Can you work these out from the model? Positions are in its coordinate system, mm. A direction names the side the tool comes from. Give positions to 0.01 mm unless a question says otherwise; leave off trailing zeros. Order: outer loops, then holes, each group sorted by start corner. A loop starts at its lowest first (then second) coordinate and runs counter-clockwise, first axis right, second up. Notation, with made-up numbers: (13.25, 55) -> (17.25, 55) arc R20 cw to (17.25, 80) -> close; hole circle Ø2 at (2, 4.25). An arc over 180 degrees is marked (long way). Answer as CSV lines item,"result".
```python
from build123d import *

# Parameters (mm, degrees)
SKETCH_R     = 1.6
PAD_DEPTH    = 3
SKETCH001_W  = 5
SKETCH001_H  = 65
PAD001_DEPTH = 2
POCKET_DEPTH = 5


with BuildPart() as part:
    # Sketch → Pad (new body)
    with BuildSketch(Plane.XY):
        Polygon((-80, 32.5), (-80, -32.5), (-35, -32.5), (-35, -15), (75, -15), (75, 15), (-35, 15), (-35, 32.5), align=None)
        with Locations((-70, 22.5)):
            Circle(SKETCH_R, mode=Mode.SUBTRACT)
        with Locations((-45, 22.5)):
            Circle(SKETCH_R, mode=Mode.SUBTRACT)
        with Locations((-70, 7.5)):
            Circle(SKETCH_R, mode=Mode.SUBTRACT)
        with Locations((-45, 7.5)):
            Circle(SKETCH_R, mode=Mode.SUBTRACT)
        with Locations((-70, -7.5)):
            Circle(SKETCH_R, mode=Mode.SUBTRACT)
        with Locations((-45, -7.5)):
            Circle(SKETCH_R, mode=Mode.SUBTRACT)
        with Locations((-70, -22.5)):
            Circle(SKETCH_R, mode=Mode.SUBTRACT)
        with Locations((-45, -22.5)):
            Circle(SKETCH_R, mode=Mode.SUBTRACT)
        with Locations((45, 7.5)):
            Circle(SKETCH_R, mode=Mode.SUBTRACT)
        with Locations((45, -7.5)):
            Circle(SKETCH_R, mode=Mode.SUBTRACT)
        with Locations((70, 7.5)):
            Circle(SKETCH_R, mode=Mode.SUBTRACT)
        with Locations((70, -7.5)):
            Circle(SKETCH_R, mode=Mode.SUBTRACT)
    extrude(amount=PAD_DEPTH)

    # Sketch001 → Pad001 (new body)
    with BuildSketch(Plane.XY.offset(3)):
        with Locations((-77.5, 0)):
            Rectangle(SKETCH001_W, SKETCH001_H)
    extrude(amount=PAD001_DEPTH)

    # Sketch002 → Pocket (cut)
    with BuildSketch(Plane.XY.offset(3)):
        with BuildLine():
            ThreePointArc((-25, 8), (-33.000002, 1e-06), (-25.000002, -8))
            Line((-25.000002, -8), (25.000002, -8))
            ThreePointArc((25.000002, -8), (33.000002, 1e-06), (25, 8))
            Line((-25, 8), (25, 8))
        make_face()
    extrude(amount=-POCKET_DEPTH, mode=Mode.SUBTRACT)


solid = part.part
```
Item 1: Please list where these lines run through material, in increasing order: line 1 along Y through (x, z) = (45, 1.5); line 2 along Y through (x, z) = (-45, 1.45); line 3 along Y through (x, z) = (-19, 2.95).
Numbers:
line 1,"y = -15 to -9.1, -5.9 to 5.9, 9.1 to 15"
line 2,"y = -32.5 to -24.1, -20.9 to -9.1, -5.9 to 5.9, 9.1 to 20.9, 24.1 to 32.5"
line 3,"y = -15 to -8, 8 to 15"
Item 2: For pin 1 (1.5 mm diameter, centred on x = -10, z = 1, fed in from +Y); pin 2 (2.5 mm diameter, centred on y = -20, z = 2, fed in from +X); pin 3 (5 mm diameter, centred on x = 45, y = 7.5, fed in from +Z), each with a flat end and sliding along its axis, tell me the tip position at first contact or that it passes through.
Numbers:
pin 1,"stops at y = 15"
pin 2,"stops at x = -35"
pin 3,"stops at z = 3"
Item 3: For faces 1 (the flat face through (21, 15, 1)), 2 (the flat face through (-35, -24, 1)), 3 (the cylindrical face through (33, 0, 2)), which set-ups out of +Z, -Z, +X, -X, +Y, -Y let a thin tool reach every point of the face, with its end or its side?
Numbers:
face 1,"+Z, -Z, +X, +Y"
face 2,"+Z, -Z, +X, -Y"
face 3,"+Z, -Z"
Item 4: We'd pull the mould along X, two halves only. Please class faces 4 (the cylindrical face through (71.526, 7.981, 1.479)), 5 (the flat face through (-80, 0, 2)), 6 (the flat face through (-58, 32.5, 1)): released by +X, released by -X, zero draft, split by the parting line, or undercut.
Numbers:
face 4,"undercut"
face 5,"released by -X"
face 6,"zero draft"
Item 5: Imagine slicing it at B-B, the plane z = 1.5. Give the number of separate pieces and of enclosed holes in the cut face, then the cut area to 3 significant figures.
Numbers:
separate pieces,"1"
enclosed holes,"13"
area,"5,130 mm²"
Item 6: Imagine slicing it at C-C, the plane y = -22.5. Please give me the cut outline in (x, z), then the cut area to 3 significant figures.
Numbers:
outline,"(-80, 0) -> (-71.6, 0) -> (-71.6, 3) -> (-75, 3) -> (-75, 5) -> (-80, 5) -> close; (-68.4, 0) -> (-46.6, 0) -> (-46.6, 3) -> (-68.4, 3) -> close; (-43.4, 0) -> (-35, 0) -> (-35, 3) -> (-43.4, 3) -> close"
area,"126 mm²"
Item 7: Imagine slicing it at A-A, the plane x = -8. Please give me the cut outline in (y, z).
Numbers:
outline,"(-15, 0) -> (-8, 0) -> (-8, 3) -> (-15, 3) -> close; (8, 0) -> (15, 0) -> (15, 3) -> (8, 3) -> close"
Item 8: Imagine slicing it at D-D, the plane x = 45. Please give me the cut outline in (y, z), then the cut area to 3 significant figures.
Numbers:
outline,"(-15, 0) -> (-9.1, 0) -> (-9.1, 3) -> (-15, 3) -> close; (-5.9, 0) -> (5.9, 0) -> (5.9, 3) -> (-5.9, 3) -> close; (9.1, 0) -> (15, 0) -> (15, 3) -> (9.1, 3) -> close"
area,"70.8 mm²"
